Work out the finished part from the listing and answer in its coordinate system (mm). Face numbers are marked on the shaded views. A direction names the side the tool comes from. Give positions to 0.01 mm unless a question says otherwise; leave off trailing zeros. Loops run counter-clockwise (first coordinate to the right, second up) from the corner with the lowest first, then second, coordinate; pieces in that order, holes last. Notation, with made-up numbers: (45.5, 10.5) -> (96.5, 10.5) arc R18 ccw to (96.5, 45.5) -> close; hole circle Ø10 at (22.5, 74.25). An arc over 180 degrees is marked (long way). Answer as CSV lines item,"result". Start each with the question number.
1. Find section C-C, the plane z = 37.5. Give the vertices of the cut face in (x, y).
2. Find section A-A, the plane x = -8. Give the vertices of the cut face in (y, z).
3. Find the intervals of material crossed by line 1 along Z through (x, y) = (7.5, 14); line 2 along X through (y, z) = (16, 34); line 3 along Y through (x, z) = (-6, 44), in increasing order.
4. Find section B-B, the plane y = 30. Give the vertices of the cut face in (x, z).
5. A tool of negligible diameter and unlimited length cuts with its end or side. For the marked faces 5 and 6, from which of +Z, -Z, +X, -X, +Y, -Y can it reach the whole face along a straight path? Write none if from no direction.
6. Flat-ended cylindrical pins translate along their axes: pin 1 Ø9.5 at (x, y) = (12.5, 18) entering from -Z; pin 2 Ø3 at (x, z) = (-11, 28) entering from +Y. Find the tip coordinate at first contact, or state that the pin passes through.
7. Determine the mould class of the marked faces 1, 2, 3 and 4 for opening direction X: +X half, -X half, draft (parallel to the pull), parting line (faces both ways), or undercut.
8. Find section D-D, the plane y = 8.5. Give the vertices of the cut face in (x, z).
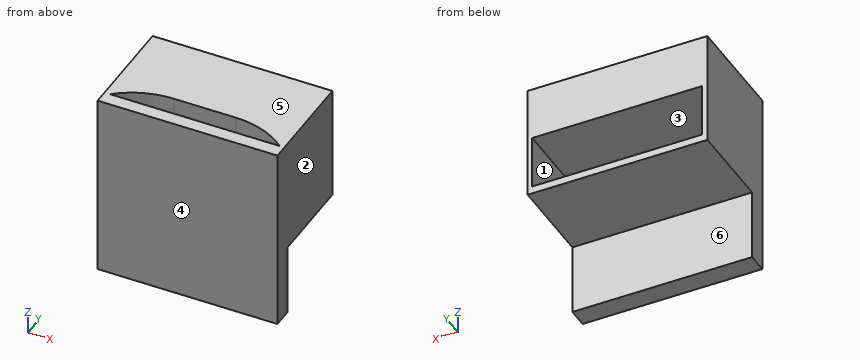
from build123d import *

# Parameters (mm, degrees)
F0_W         = 63.5
F0_H         = 63.5
F1_DEPTH     = 38.1
F2_DEPTH     = 58.42
F3_W         = 60
F3_H         = 7
F4_DEPTH     = 38.1
F5_W         = 60
F5_H         = 19.05
F6_DEPTH     = 50.8
F7_DEPTH     = 25.4
F8_W         = 38.1
F8_H         = 17.6288653165
F9_DEPTH     = 76.2
F10_T1_DEPTH = 19.05
F11_W        = 63.5
F11_H        = 13.4413276523
F12_DEPTH    = 25.4
F13_DEPTH    = 6.35


# Not quite as in the source:
# - a fillet or chamfer that OpenCascade refuses, or shapes differently, is made with other operations: its cross-section is extruded or revolved along the edge and cut away or added


with BuildPart() as f1:
    # F0 (on Top) → F1 (new body)
    with BuildSketch(Plane.XY):
        with Locations((-0.7267157435, 4.9544320554)):
            Rectangle(F0_W, F0_H)
    extrude(amount=F1_DEPTH)

    # F0 (on Top) → F2 (join)
    with BuildSketch(Plane.XY):
        with Locations((-0.7267157435, 4.9544320554)):
            Rectangle(F0_W, F0_H)
    extrude(amount=F2_DEPTH)

    # F3 (on face) → F4 (cut)
    with BuildSketch(Plane.XY.offset(58.42)):
        with Locations((-0.5849367008, 6.9008102814)):
            Rectangle(F3_W, F3_H)
    extrude(amount=-F4_DEPTH, mode=Mode.SUBTRACT)

    # F5 (on face) → F6 (cut)
    with BuildSketch(Plane.XZ.offset(-10.4008102814)):
        with Locations((-0.5849367008, 29.845)):
            Rectangle(F5_W, F5_H)
    extrude(amount=-F6_DEPTH, mode=Mode.SUBTRACT)

    # F7 (cut): a face of the model
    f7_faces = [f1.faces().sort_by_distance(p)[0] for p in [
        (-0.7267157435, -26.7955679446, 29.21),
    ]]
    extrude(f7_faces, amount=-F7_DEPTH, mode=Mode.SUBTRACT)

    # F8 (on face) → F9 (cut)
    with BuildSketch(Plane.YZ.offset(31.0232842565)):
        with Locations((17.6544320554, 8.8144326583)):
            Rectangle(F8_W, F8_H)
    extrude(amount=-F9_DEPTH, mode=Mode.SUBTRACT)

    # F10: fillet of radius 29.4340917525 on 2 edges, made by hand

    # F10_s2 → F10_t1 (join)
    with BuildSketch(Plane.XY.offset(39.37)):
        with BuildLine():
            ThreePointArc((29.4150632992, 3.4008102814), (20.5103197353, 8.5954433667), (10.3604763309, 10.4008102814))
            Line((10.3604763309, 10.4008102814), (29.4150632992, 10.4008102814))
            Line((29.4150632992, 10.4008102814), (29.4150632992, 3.4008102814))
        make_face()
        with BuildLine():
            ThreePointArc((-30.5849367008, 3.4008102814), (-21.6801931368, 8.5954433667), (-11.5303497324, 10.4008102814))
            Line((-11.5303497324, 10.4008102814), (-30.5849367008, 10.4008102814))
            Line((-30.5849367008, 10.4008102814), (-30.5849367008, 3.4008102814))
        make_face()
    extrude(amount=F10_T1_DEPTH)

    # F11 (on face) → F12 (join)
    with BuildSketch(Plane(origin=(0, 0, 17.6288653165), x_dir=(1, 0, 0), z_dir=(0, 0, -1))):
        with Locations((-0.7267157435, -5.3250958815)):
            Rectangle(F11_W, F11_H)
    extrude(amount=F12_DEPTH)

    # F13 (cut): a face of the model
    f13_faces = [f1.faces().sort_by_distance(p)[0] for p in [
        (-0.7267157435, 12.0457597077, 4.9288653165),
    ]]
    extrude(f13_faces, amount=-F13_DEPTH, mode=Mode.SUBTRACT)


solid = f1.part
Resolved:
1,outline,"(-32.48, -1.4) -> (31.02, -1.4) -> (31.02, 36.7) -> (29.42, 36.7) -> (29.42, 3.4) -> (-30.58, 3.4) -> (-30.58, 36.7) -> (-32.48, 36.7) -> close"
2,outline,"(-1.4, -7.77) -> (5.7, -7.77) -> (5.7, 17.63) -> (36.7, 17.63) -> (36.7, 20.32) -> (3.4, 20.32) -> (3.4, 58.42) -> (-1.4, 58.42) -> close; (10.4, 39.37) -> (36.7, 39.37) -> (36.7, 58.42) -> (10.4, 58.42) -> close"
3,line 1,"z = 17.63 to 20.32, 39.37 to 58.42"
3,line 2,"x = -32.48 to -30.58, 29.42 to 31.02"
3,line 3,"y = -1.4 to 3.4, 10.4 to 36.7"
4,outline,"(-32.48, 17.63) -> (31.02, 17.63) -> (31.02, 58.42) -> (-32.48, 58.42) -> close; hole (-30.58, 20.32) -> (29.42, 20.32) -> (29.42, 39.37) -> (-30.58, 39.37) -> close"
5,face 5,"+Z, +X, -X, +Y, -Y"
5,face 6,"-Z, +X, -X, +Y"
6,pin 1,"stops at z = 17.63"
6,pin 2,"stops at y = 3.4"
7,face 1,"undercut"
7,face 2,"+X half"
7,face 3,"undercut"
7,face 4,"draft"
8,outline,"(-32.48, 17.63) -> (31.02, 17.63) -> (31.02, 58.42) -> (20.77, 58.42) -> (20.77, 39.37) -> (29.42, 39.37) -> (29.42, 20.32) -> (-30.58, 20.32) -> (-30.58, 39.37) -> (-21.94, 39.37) -> (-21.94, 58.42) -> (-32.48, 58.42) -> close"
